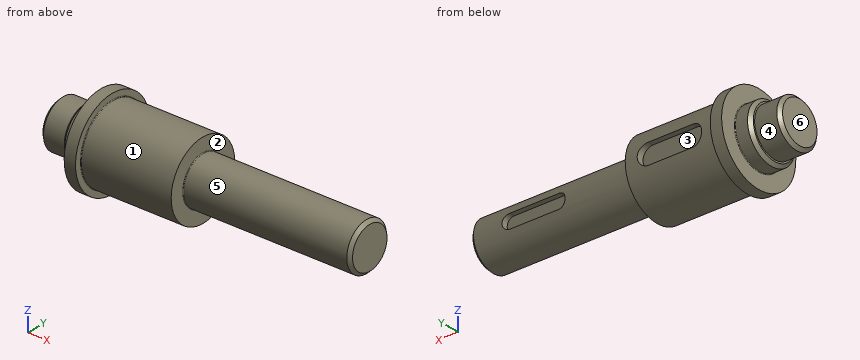
```python
from build123d import *

# Parameters (mm, degrees)
CUT_EXTRUDE_1_DEPTH      = 11
CUT_EXTRUDE_2_DEPTH      = 359.209373116
CUT_EXTRUDE_2_DEPTH_BACK = 1
CHAMFER_1_SIZE           = 5
FILLET_1_R               = 1


with BuildPart() as part:
    # 草图1 → 旋转1 (revolve)
    with BuildSketch(Plane.XY, mode=Mode.PRIVATE) as revolve_1_sk:
        Polygon((-152.788338001, 0), (-152.788338001, 37.5), (-112.788338001, 37.5), (-112.788338001, 45), (-87.788338001, 45), (-87.788338001, 70), (-69.788338001, 70), (-69.788338001, 60), (73.211661999, 60), (73.211661999, 37.5), (337.211661999, 37.5), (337.211661999, 0), align=None)
    revolve(revolve_1_sk.sketch.rotate(Axis((-105.28115942, 0, 0), (1, 0, 0)), 90), axis=Axis((-105.28115942, 0, 0), (1, 0, 0)))

    # 草图2 → 切除-拉伸1 (cut)
    with BuildSketch(Plane(origin=(0, 60, 0), x_dir=(-1, 0, 0), z_dir=(0, 1, 0))):
        with BuildLine():
            Line((-38.211661999, 15.832796851), (31.788338001, 15.832796851))
            ThreePointArc((31.788338001, 15.832796851), (47.788338001, -0.167203149), (31.788338001, -16.167203149))
            Line((31.788338001, -16.167203149), (-38.211661999, -16.167203149))
            ThreePointArc((-38.211661999, -16.167203149), (-54.211661999, -0.167203149), (-38.211661999, 15.832796851))
        make_face()
    extrude(amount=-CUT_EXTRUDE_1_DEPTH, mode=Mode.SUBTRACT)

    # 草图3 → 切除-拉伸2 (cut, two sides: drawn at the far end of the back side and taken through both)
    with BuildSketch(Plane(origin=(0, 28.5, 0), x_dir=(-1, 0, 0), z_dir=(0, 1, 0)).offset(-CUT_EXTRUDE_2_DEPTH_BACK)):
        with BuildLine():
            Line((-198.211661999, 11), (-276.211661999, 11))
            ThreePointArc((-276.211661999, 11), (-287.227527816, -0.015865818), (-276.211661999, -11.031731635))
            Line((-276.211661999, -11.031731635), (-198.211661999, -11.031731635))
            ThreePointArc((-198.211661999, -11.031731635), (-187.195796181, -0.015865818), (-198.211661999, 11))
        make_face()
    extrude(amount=CUT_EXTRUDE_2_DEPTH + CUT_EXTRUDE_2_DEPTH_BACK, mode=Mode.SUBTRACT)

    # 倒角1
    chamfer_1_edges = [part.edges().sort_by_distance(p)[0] for p in [
        (-112.788338001, 0, -45),
        (-152.788338001, 0, -37.5),
        (337.211661999, 0, -37.5),
    ]]
    chamfer(chamfer_1_edges, length=CHAMFER_1_SIZE)

    # 圆角1
    fillet_1_edges = [part.edges().sort_by_distance(p)[0] for p in [
        (-69.788338001, 0, -60),
        (-87.788338001, 0, -45),
        (73.211661999, 0, -37.5),
    ]]
    fillet(fillet_1_edges, radius=FILLET_1_R)


solid = part.part
```
Could you check a few things on this model? Use its own coordinates, in mm. Face numbers are marked on the shaded views. A direction names the side the tool comes from. Give positions to 0.01 mm unless a question says otherwise; leave off trailing zeros. Write each loop counter-clockwise with the first axis right and the second up, starting at its lowest first coordinate (ties: lowest second). Pieces come first, ordered by that corner, then holes. Notation, with made-up numbers: (52, 74) -> (75, 74) arc R19 cw to (75, 91) -> close; hole circle Ø7 at (29.5, -6.5). An arc over 180 degrees is marked (long way). Write each question's results on one line, items separated by ' | '.
1. I need wall thicknesses on L1, parallel to X at y = 39, z = -4; L2, parallel to X at y = -54, z = -26; L3, parallel to Y at x = 245, z = -2. Which ranges of each line are inside material? Lowest first, please.
Check sheet entries:
L1: x = -112.79 to 73.21 | L2: x = -87.79 to 73.21 | L3: y = -37.45 to 27.5
2. Will these pins go through, and if not, where does the flat tip stop? pin 1 Ø3 at (y, z) = (-38.5, -32.5) entering from -X; pin 2 Ø6 at (x, z) = (34.5, 1) entering from +Y; pin 3 Ø10 at (x, y) = (14, 54.5) entering from -Z.
Check sheet entries:
pin 1: stops at x = -87.79 | pin 2: stops at y = 49 | pin 3: stops at z = -33.91
3. I want a section at C-C, the plane x = -96. Write out the boundary of the cut face in (y, z), then the cut area to 3 significant figures.
Check sheet entries:
outline: circle Ø90 at (0, 0) | area: 6,360 mm²
4. I want a section at D-D, the plane x = 209. Write out the boundary of the cut face in (y, z), then the cut area to 3 significant figures.
Check sheet entries:
outline: (27.5, -11.03) -> (27.5, 11) -> (35.85, 11) arc R37.5 ccw (long way) to (35.84, -11.03) -> close | area: 4,210 mm²
5. If we mould it in two halves opening along Z, with no side actions, what happens to the marked faces 1, 2 and 3? For each: released by +Z, released by -Z, zero draft, split by the parting line, or undercut.
Check sheet entries:
face 1: split by the parting line | face 2: zero draft | face 3: undercut
6. I want a section at B-B, the plane x = -16.5. Write out the boundary of the cut face in (y, z), then the cut area to 3 significant figures.
Check sheet entries:
outline: (49, -16.17) -> (49, 15.83) -> (57.87, 15.83) arc R60 ccw (long way) to (57.78, -16.17) -> close | area: 11,000 mm²
7. On a 3-axis mill with a long thin cutter (end or side, diameter ignored), from which of +Z, -Z, +X, -X, +Y, -Y can I reach the whole of each face in a straight line? I mean the marked faces 4, 5 and 6. Say none if no direction works.
Check sheet entries:
face 4: -X | face 5: +X | face 6: +Z, -Z, -X, +Y, -Y
